Source: CAD feature listing. Evaluate the final solid. Frame: model axes, mm. Face numbers are marked on the shaded views. A direction names the side the tool comes from. Round coordinates to 2 decimals unless told otherwise and drop trailing zeros. Order: outer loops, then holes, each group sorted by start corner. A loop starts at its lowest first (then second) coordinate and runs counter-clockwise, first axis right, second up. Notation, with made-up numbers: (36, 26.25) -> (65, 26.25) arc R25 ccw to (65, 56.25) -> close; hole circle Ø3 at (40, 73.5). An arc over 180 degrees is marked (long way). One line per item, written item: value. Start each with the question number.
1) Pin query (flat end, axial travel): P1, Ø1, axis at x = -31, z = 13, coming from the -Y side; P2, Ø6, axis at y = -1.5, z = 7.5, coming from the +X side; P3, Ø3.5, axis at y = 0.5, z = 20, coming from the +X side. Return the tip coordinate at first contact, or that it passes through.
2) Reachability of the marked faces 1, 2, 3, 4 and 5 from +Z, -Z, +X, -X, +Y, -Y: full face, straight path, thin tool, end or side. Return the list, or none.
3) Section A-A (y = -10). Return the cut outline in (x, z).
4) Section D-D (x = 7). Return the cut outline in (y, z), and give its area (3 significant figures).
5) Ray query, L1, parallel to X at y = -1.5, z = 20; L2, parallel to X at y = -3, z = 11; L3, parallel to Y at x = -32.5, z = 26.5. Return the intervals inside material, ascending.
6) Section B-B (y = -4.75). Return the cut outline in (x, z), and give its area (3 significant figures).
7) Mould query, pull axis X, two halves, no side actions, for the marked faces 6, 7 and 8. Classes: pulls with the +X half, pulls with the -X half, needs draft (parallel to the pull), parting line crosses it, or undercut.
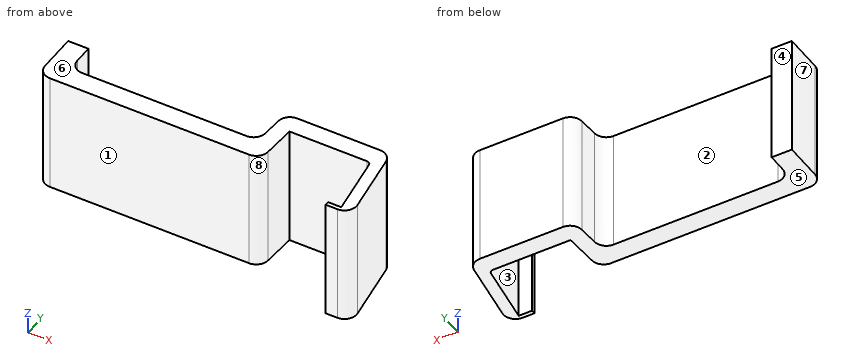
```python
from build123d import *

# Parameters (mm, degrees)
F1_DEPTH  = 30
F1_FACE_W = 0.99785
F1_FACE_H = 30
F2_DEPTH  = 3


with BuildPart() as f1:
    # F0 (on Top) → F1 (new body)
    with BuildSketch(Plane.XY):
        with BuildLine():
            ThreePointArc((-50.862886, -7.958589), (-49.984207, -10.07991), (-47.862886, -10.958589))
            Line((-47.862886, -10.958589), (1.29883, -10.958589))
            ThreePointArc((1.29883, -10.958589), (3.360601, -10.137833), (4.29423, -8.124658))
            Line((4.29423, -8.124658), (4.73644, -0.148474))
            Line((4.73644, -0.148474), (4.744672, 0))
            Line((4.744672, 0), (9.380593, 0))
            Line((9.380593, 0), (23.877159, 0))
            ThreePointArc((23.877159, 0), (24.532454, -0.244627), (24.867143, -0.858825))
            Line((24.867143, -0.858825), (27.003476, -15.839754))
            Line((27.003476, -15.839754), (26.708684, -15.839754))
            Line((26.708684, -15.839754), (26.708684, -16.837603))
            ThreePointArc((26.708684, -16.837603), (28.898037, -15.762383), (29.565059, -13.416228))
            Line((29.565059, -13.416228), (27.37089, 1.970275))
            ThreePointArc((27.37089, 1.970275), (26.366823, 3.812867), (24.400936, 4.546749))
            Line((24.400936, 4.546749), (3.933248, 4.546749))
            ThreePointArc((3.933248, 4.546749), (1.871477, 3.725993), (0.937848, 1.712818))
            Line((0.937848, 1.712818), (0.669652, -3.124658))
            ThreePointArc((0.669652, -3.124658), (-0.263978, -5.137833), (-2.325748, -5.958589))
            Line((-2.325748, -5.958589), (-42.862886, -5.958589))
            ThreePointArc((-42.862886, -5.958589), (-44.984207, -5.07991), (-45.862886, -2.958589))
            Line((-45.862886, -2.958589), (-45.862886, 1.602761))
            Line((-45.862886, 1.602761), (-50.862886, 1.602761))
            Line((-50.862886, 1.602761), (-50.862886, -7.958589))
        make_face()
    extrude(amount=F1_DEPTH)

    # F1_face (on face) → F2 (join)
    with BuildSketch(Plane(origin=(26.708684, -16.338679, 15), x_dir=(0, -1, 0), z_dir=(-1, 0, 0))):
        Rectangle(F1_FACE_W, F1_FACE_H)
    extrude(amount=F2_DEPTH)


solid = f1.part
```
Findings:
1. P1: y = -10.96
1. P2: x = 28.29
1. P3: x = 27.83
2. face 1: +Z, -Z, -X, -Y
2. face 2: +Z, -Z, +Y
2. face 3: +Z, -Z
2. face 4: +Z, -Z, -X, +Y
2. face 5: -Z, +X, -X, +Y, -Y
3. outline: (-50.06, 0) -> (3.5, 0) -> (3.5, 30) -> (-50.06, 30) -> close; (26.17, 0) -> (29.08, 0) -> (29.08, 30) -> (26.17, 30) -> close
4. outline: (0, 0) -> (4.55, 0) -> (4.55, 30) -> (0, 30) -> close
4. area: 136 mm2
5. L1: -50.86 to -45.86, 0.76 to 4.66, 24.96 to 27.87
5. L2: -50.86 to -45.86, 0.68 to 4.58, 25.17 to 28.08
5. L3: -10.96 to -5.96
6. outline: (-50.86, 0) -> (-45.27, 0) -> (-45.27, 30) -> (-50.86, 30) -> close; (0.08, 0) -> (4.48, 0) -> (4.48, 30) -> (0.08, 30) -> close; (25.42, 0) -> (28.33, 0) -> (28.33, 30) -> (25.42, 30) -> close
6. area: 387 mm2
7. face 6: needs draft
7. face 7: pulls with the -X half
7. face 8: undercut
